Autodesk Inventor part; units mm, degrees
ref_plane "YZ Plane" through (0, 0, 0) normal (1, 0, 0) x (0, 1, 0)
ref_plane "XZ Plane" through (0, 0, 0) normal (0, 1, 0) x (-1, 0, 0)
ref_plane "XY Plane" through (0, 0, 0) normal (0, 0, 1) x (1, 0, 0)
sketch "Sketch1" plane through (0, 0, 0) normal (0, 0, 1) x (1, 0, 0)
  circle A0 centre (0, 0) radius 7.5
  line L0 (-17.5, 0) -> (-7.5, 0)
  line L1 (7.5, 0) -> (17.5, 0)
  line L2 (-17.5, 0) -> (-17.5, 10.5)
  line L3 (-17.5, 10.5) -> (17.5, 10.5)
  line L4 (17.5, 10.5) -> (17.5, 0)
  dimension "d5" = 15
  dimension "d6" = 0
  dimension "d8" = 0
  dimension "d11" = 10
  dimension "d13" = 10
  dimension "d19" = 10.5
  dimension "d64" = 35
extrude "Extrusion1" add sketch "Sketch1" along normal blind 48 contours A0 L0 L2 L3 L4 L1
sketch "Sketch3" plane through (7.5, 0, 0) normal (0, -1, 0) x (1, 0, 0)
  line L0 (10, 0) -> (10, 48)
  line L1 (0, 48) -> (10, 48)
  line L2 (0, 0) -> (0, 48)
  line L3 (0, 0) -> (10, 0)
  line L4 (-25, 0) -> (-15, 0)
  line L5 (-15, 0) -> (-15, 48)
  line L6 (-25, 48) -> (-15, 48)
  line L7 (-25, 0) -> (-25, 48)
  point P0 (-7.5, 0)
  point P1 (5, 4.5)
  point P2 (5, 24)
  point P3 (5, 43.5)
  point P4 (-20, 43.5)
  point P5 (-20, 4.5)
  point P6 (-20, 24)
  dimension "d31" = 48
  dimension "d35" = 5
  dimension "d44" = 4.5
  dimension "d45" = 4.5
  dimension "d46" = 24
  dimension "d47" = 5
  dimension "d48" = 10
  dimension "d49" = 10
hole "Hole1" at (12.5, 0, 4.5) at (12.5, 0, 24) at (12.5, 0, 43.5) at (-12.5, 0, 43.5) at (-12.5, 0, 4.5) at (-12.5, 0, 24) direction (0, 1, 0) diameter 3 end through all
chamfer "Chamfer1" distance 3 angle 45 4 edges at (17.5, 5.25, 48) (-17.5, 5.25, 48) (-17.5, 5.25, 0) (17.5, 5.25, 0)
fillet "Fillet2" radius 2 8 edges at (14.5, 5.25, 48) (17.5, 5.25, 45) (17.5, 5.25, 3) (14.5, 5.25, 0) (-14.5, 5.25, 0) (-17.5, 5.25, 3) (-17.5, 5.25, 45) (-14.5, 5.25, 48)
sketch "Sketch4" plane through (17.5, 0, 3.8284) normal (1, 0, 0) x (0, 0, -1)
  line L0 (0, 10.5) -> (-40.3431, 10.5)
  line L1 (3.8284, 0) -> (3.8284, 10.5)
  line L2 (-44.1716, 10.5) -> (-44.1716, 0)
  point P0 (-10.4216, 7.3)
  point P1 (-29.9216, 7.3)
  dimension "d54" = 3.2
  dimension "d55" = 14.25
  dimension "d56" = 14.25
hole "Hole2" at (17.5, 7.3, 14.25) at (17.5, 7.3, 33.75) direction (-1, 0, 0) diameter 2.5 depth 10 tip angle 118
equation "\"d13\" = d11"
properties part number "3DP_PLA_X_end_bottom_half" material "ABS Plastic"
Model file for the job. Use its own axes, mm. A direction names the side the tool comes from. Give positions to 0.01 mm unless a question says otherwise; leave off trailing zeros. Order: outer loops, then holes, each group sorted by start corner. A loop starts at its lowest first (then second) coordinate and runs counter-clockwise, first axis right, second up.
1) Saw through at A-A, the plane x = -12.5. Write the cut outline in (y, z).
2) Wall check: probe 1 along X at (y, z) = (7.75, 24); probe 2 along Z at (x, y) = (12.5, 4.25); probe 3 along X at (y, z) = (2, 4.5). Give the ranges that are in metal, low to high.
3) Pin check, flat tips, straight feed: pin 1 (5 mm diameter, centred on x = 1.5, z = 9.5, fed in from -Y); pin 2 (2 mm diameter, centred on y = 7.3, z = 14.25, fed in from +X). Stop position of each tip, or through.
4) Saw through at C-C, the plane z = 4.5. Write the cut outline in (x, y).
5) Saw through at D-D, the plane z = 40.5. Write the cut outline in (x, y), then the cut area to 3 significant figures.
6) 3-axis set-ups, long thin cutter, end or side, ignore diameter. For faces 4 (the flat face through (-16, 5.2, 1.5)), 5 (the cylindrical face through (12.43, 8.06, 15.24)): which of +Z, -Z, +X, -X, +Y, -Y reach the whole face in a straight line?
7) Saw through at B-B, the plane y = 1. Write the cut outline in (x, z), then the cut area to 3 significant figures.
8) Mould opens along Y. For faces 1 (the cylindrical face through (-17.35, 5.32, 44.93)), 2 (the cylindrical face through (12.43, 8.409, 33.173)), 3 (the cylindrical face through (-0.16, 7.5, 23.66)) say: +Y half, -Y half, draft (parallel to the pull), parting line (faces both ways), or undercut.
Computed:
1. outline: (0, 0) - (10.5, 0) - (10.5, 3) - (0, 3) - close; (0, 6) - (10.5, 6) - (10.5, 22.5) - (0, 22.5) - close; (0, 25.5) - (10.5, 25.5) - (10.5, 42) - (0, 42) - close; (0, 45) - (10.5, 45) - (10.5, 48) - (0, 48) - close
2. probe 1: x = -17.5 to -14, -11 to 11, 14 to 17.5
2. probe 2: z = 0 to 3, 6 to 22.5, 25.5 to 42, 45 to 48
2. probe 3: x = -17.5 to -14, -11 to -7.23, 7.23 to 11, 14 to 17.5
3. pin 1: stops at y = 6.34
3. pin 2: stops at x = 7.35
4. outline: (-17.5, 0) - (-14, 0) - (-14, 10.5) - (-17.5, 10.5) - close; (-11, 0) - (-7.5, 0) arc R7.5 cw to (7.5, 0) - (11, 0) - (11, 10.5) - (-11, 10.5) - close; (14, 0) - (17.5, 0) - (17.5, 10.5) - (14, 10.5) - close
5. outline: (-17.5, 0) - (-7.5, 0) arc R7.5 cw to (7.5, 0) - (17.5, 0) - (17.5, 10.5) - (-17.5, 10.5) - close
5. area: 279 mm2
6. face 4: -Z, -X, +Y, -Y
6. face 5: +X
7. outline: (-17.5, 3.83) arc R2 ccw to (-16.91, 2.41) - (-15.09, 0.59) arc R2 ccw to (-13.67, 0) - (-7.43, 0) - (-7.43, 48) - (-13.67, 48) arc R2 ccw to (-15.09, 47.41) - (-16.91, 45.59) arc R2 ccw to (-17.5, 44.17) - close; (7.43, 0) - (13.67, 0) arc R2 ccw to (15.09, 0.59) - (16.91, 2.41) arc R2 ccw to (17.5, 3.83) - (17.5, 44.17) arc R2 ccw to (16.91, 45.59) - (15.09, 47.41) arc R2 ccw to (13.67, 48) - (7.43, 48) - close; hole circle Ø3 at (-12.5, 4.5); hole circle Ø3 at (-12.5, 24); hole circle Ø3 at (-12.5, 43.5); hole circle Ø3 at (12.5, 4.5); hole circle Ø3 at (12.5, 24); hole circle Ø3 at (12.5, 43.5)
7. area: 905 mm2
8. face 1: draft
8. face 2: undercut
8. face 3: -Y half
